```python
from build123d import *

# Parameters (mm, degrees)
F0_R     = 17.4
F1_DEPTH = 25
F3_DEPTH = 50


# Not quite as in the source:
# - ends of sketch curves that miss each other by under 0.0002 mm in the source are joined


with BuildPart() as f1:
    # F0 (on Front) → F1 (new body)
    with BuildSketch(Plane.XZ):
        with BuildLine():
            ThreePointArc((-19.4763321764, 4.5467004469), (0, 20), (19.4763321764, 4.5467004469))
            Line((19.4763321764, 4.5467004469), (12.5, 34.4306491315))
            Line((12.5, 34.4306491315), (0, 34.4306491315))
            Line((0, 34.4306491315), (-12.5, 34.4306491315))
            Line((-12.5, 34.4306491315), (-19.4763321764, 4.5467004469))
        make_face()
        with BuildLine():
            ThreePointArc((-19.9999883661, -0.0215721294), (0.0107860663, -19.9999970915), (20, 0))
            ThreePointArc((20, 0), (19.8686517349, 2.2883789537), (19.4763321764, 4.5467004469))
            ThreePointArc((19.4763321764, 4.5467004469), (0, 20), (-19.4763321764, 4.5467004469))
            ThreePointArc((-19.4763321764, 4.5467004469), (-19.8686517349, 2.2883789537), (-20, 0))
            ThreePointArc((-20, 0), (-19.9999970915, -0.0107860663), (-19.9999883661, -0.0215721294))
        make_face()
        Circle(F0_R, mode=Mode.SUBTRACT)
        with BuildLine():
            ThreePointArc((45, -25), (27.3223304703, -17.6776695297), (20, 0))
            ThreePointArc((20, 0), (0.0107860663, -19.9999970915), (-19.9999883661, -0.0215721294))
            ThreePointArc((-19.9999883661, -0.0215721294), (-27.3583172251, -17.7351553161), (-45.1016823096, -25.0213653552))
            Line((-45.1016823096, -25.0213653552), (-50.3546064898, -25))
            Line((-50.3546064898, -25), (-75.3500018494, -25))
            Line((-75.3500018494, -25), (-75.3500018494, -28))
            Line((-75.3500018494, -28), (74.6500011308, -28))
            Line((74.6500011308, -28), (74.65, -25))
            Line((74.65, -25), (50.3546064898, -25))
            Line((50.3546064898, -25), (45, -25))
        make_face()
    extrude(amount=F1_DEPTH)

    # F2 (on face) → F3 (cut)
    with BuildSketch(Plane.XY.offset(34.4306491315)):
        with BuildLine():
            ThreePointArc((2.25, -12.5), (1.5909902577, -10.9090097423), (0, -10.25))
            ThreePointArc((0, -10.25), (-1.5909902577, -14.0909902577), (2.25, -12.5))
        make_face()
    extrude(amount=-F3_DEPTH, mode=Mode.SUBTRACT)


solid = f1.part
```
Work out the finished part from the listing and answer in its coordinate system (mm). A direction names the side the tool comes from. Round coordinates to 2 decimals unless told otherwise and drop trailing zeros. Write each loop counter-clockwise with the first axis right and the second up, starting at its lowest first coordinate (ties: lowest second). Pieces come first, ordered by that corner, then holes.
1) Which of the six approach directions +Z, -Z, +X, -X, +Y, -Y give full straight-line access (tool end or side, diameter ignored) to faces 4 (the face through (60, -12, -25)), 5 (the face through (5, -25, -17)), 6 (the face through (-63, -12, -25))?
2) Determine the mould class of faces 1 (the face through (74.65, -12, -27)), 2 (the face through (-3.772, -12.325, -16.986)), 3 (the face through (-1, -12, -28)) for opening direction X: pulls with the +X half, pulls with the -X half, needs draft (parallel to the pull), parting line crosses it, or undercut.
3) A cutting plane is placed at C-C on x = 53.5. Determine the outline of the cut face in (y, z).
4) Flat-ended cylindrical pins translate along their axes: P1, Ø5, axis at y = -16.5, z = -20.5, coming from the -X side; P2, Ø12.5, axis at x = -61, y = -9, coming from the +Z side; P3, Ø1.5, axis at x = -36.5, y = -11.5, coming from the +Z side. Find the tip coordinate at first contact, or state that the pin passes through.
5) Consider probe 1 along Z at (x, y) = (69.5, -3.5); probe 2 along X at (y, z) = (-1.25, 5); probe 3 along X at (y, z) = (-12.5, 27.75). Determine where each line is inside the solid, lowest interval first.
6) A cutting plane is placed at D-D on z = 30. Determine the outline of the cut face in (x, y).
7) A cutting plane is placed at B-B on z = -13. Determine the outline of the cut face in (x, y).
Entries:
1. face 4: +Z, +X, +Y, -Y
1. face 5: +Z, -Z, +X, -X, -Y
1. face 6: +Z, -X, +Y, -Y
2. face 1: pulls with the +X half
2. face 2: undercut
2. face 3: needs draft
3. outline: (-25, -28) - (0, -28) - (0, -25) - (-25, -25) - close
4. P1: stops at x = -35.15
4. P2: stops at z = -25
4. P3: stops at z = -23.25
5. probe 1: z = -28 to -25
5. probe 2: x = -19.37 to -16.67, 16.67 to 19.37
5. probe 3: x = -14.06 to -2.25, 2.25 to 14.06
6. outline: (-13.53, -25) - (13.53, -25) - (13.53, 0) - (-13.53, 0) - close; hole circle Ø4.5 at (0, -12.5)
7. outline: (-23.63, -25) - (-11.57, -25) - (-11.57, 0) - (-23.63, 0) - close; (11.57, -25) - (23.65, -25) - (23.65, 0) - (11.57, 0) - close
